For this review, use the dimensioned drawing (mm, ordinates from the lowest corner) and the shaded views. A direction names the side the tool comes from. Coordinates: 2 decimals unless noted, no trailing zeros. Write each loop counter-clockwise with the first axis right and the second up, starting at its lowest first coordinate (ties: lowest second). Pieces come first, ordered by that corner, then holes.
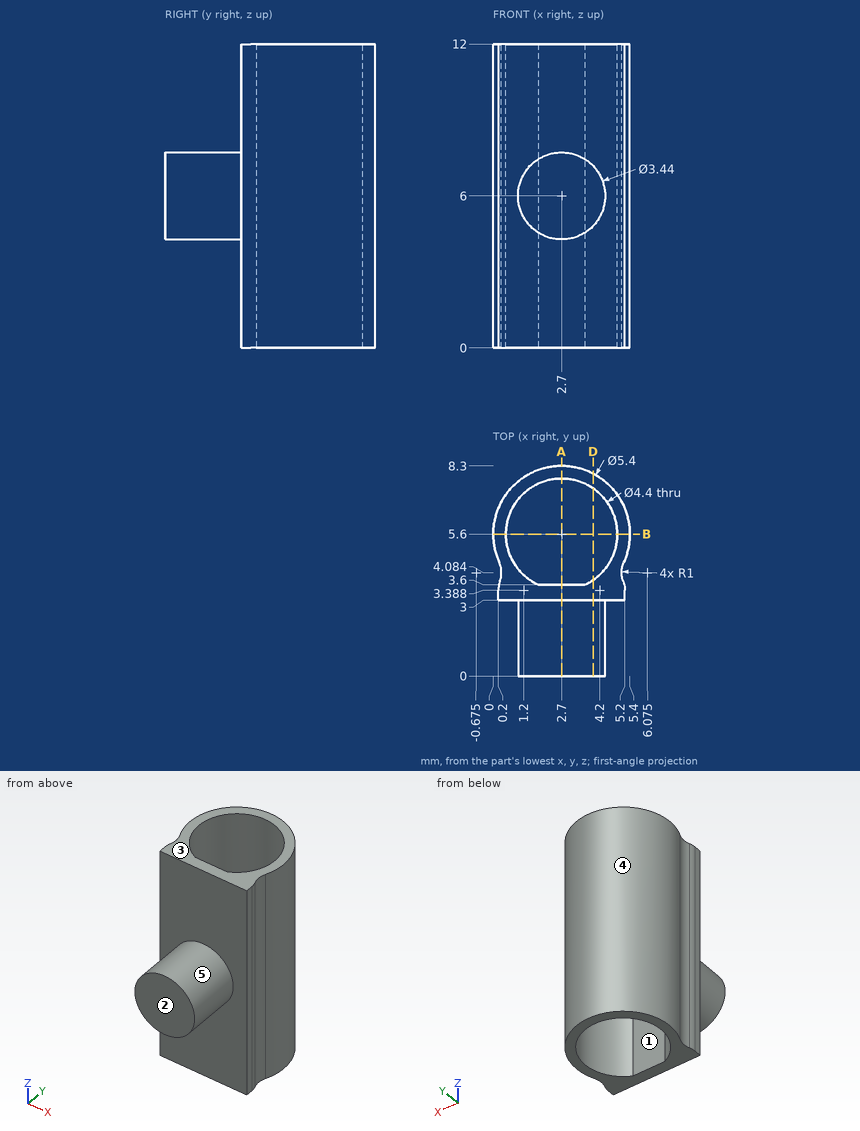
Item 1: Machinability: for the marked faces 4 and 5, which of the approach directions +Z, -Z, +X, -X, +Y, -Y give a long, thin tool a straight path to every point of the face, cutting with its end or side? Answer none if there is none.
Solved:
face 4: +Z, -Z
face 5: -Y
Item 2: Take a section at A-A, the plane x = 2.7. Write out the cut boundary in (y, z), plus the area to 3 significant figures.
Solved:
outline: (0, 4.28) - (3, 4.28) - (3, 0) - (3.6, 0) - (3.6, 12) - (3, 12) - (3, 7.72) - (0, 7.72) - close; (7.8, 0) - (8.3, 0) - (8.3, 12) - (7.8, 12) - close
area: 23.5 mm2
Item 3: Mouldability with a two-part tool opening along Y and no side actions: class the marked faces 1, 2 and 3 as pulls with the +Y half, pulls with the -Y half, needs draft (parallel to the pull), parting line crosses it, or undercut.
Solved:
face 1: undercut
face 2: pulls with the -Y half
face 3: needs draft
Item 4: Take a section at B-B, the plane y = 5.6. Write out the cut boundary in (x, z), plus the area to 3 significant figures.
Solved:
outline: (0, 0) - (0.5, 0) - (0.5, 12) - (0, 12) - close; (4.9, 0) - (5.4, 0) - (5.4, 12) - (4.9, 12) - close
area: 12.0 mm2
Item 5: Take a section at D-D, the plane x = 3.95. Write out the cut boundary in (y, z).
Solved:
outline: (0, 4.82) - (3, 4.82) - (3, 0) - (3.79, 0) - (3.79, 12) - (3, 12) - (3, 7.18) - (0, 7.18) - close; (7.41, 0) - (7.99, 0) - (7.99, 12) - (7.41, 12) - close
Item 6: To check wall thickness, follow line 1 along Y through (x, z) = (2.7, 4.5); line 2 along Y through (x, z) = (2.7, 8.5); line 3 along X through (y, z) = (5.6, 9.25). State the ranges of each line that lie inside material, in increasing order.
Solved:
line 1: y = 0 to 3.6, 7.8 to 8.3
line 2: y = 3 to 3.6, 7.8 to 8.3
line 3: x = 0 to 0.5, 4.9 to 5.4
Item 7: For pin 1 (4 mm diameter, centred on y = 1.5, z = 4.5, fed in from +X); pin 2 (1.5 mm diameter, centred on y = 3, z = 8, fed in from -X); pin 3 (3 mm diameter, centred on x = 4.5, z = 8, fed in from +Y), all flat-tipped, find the tip position at first contact; note any pin that passes through.
Solved:
pin 1: stops at x = 5.2
pin 2: stops at x = 0.2
pin 3: stops at y = 8.28
